from build123d import *

# Parameters (mm, degrees)
SKETCH1_R                       = 19.5
BOSS_EXTRUDE1_DEPTH             = 42
SKETCH2_R                       = 4.75
CUT_EXTRUDE1_DEPTH              = 3
BOSS_EXTRUDE2_DEPTH             = 22
TAP_DRILL_FOR_M4X0_7_TAP1_D     = 3.3
TAP_DRILL_FOR_M4X0_7_TAP1_DEPTH = 10.0000054
TAP_DRILL_FOR_M4X0_7_TAP1_TIP   = 0.991420021
SKETCH6_R                       = 3.5
CUT_EXTRUDE2_DEPTH              = 1.33


with BuildPart() as part:
    # Sketch1 → Boss-Extrude1 (new, symmetric)
    with BuildSketch(Plane(origin=(0, 0, 0), x_dir=(0, 0, -1), z_dir=(1, 0, 0))):
        with Locations(Location((0, 0, 0), (0, 0, 180))):
            Circle(SKETCH1_R)
    extrude(amount=BOSS_EXTRUDE1_DEPTH, both=True)

    # Sketch2 → Cut-Extrude1 (cut)
    with BuildSketch(Plane(origin=(42, 0, 0), x_dir=(0, 0, -1), z_dir=(1, 0, 0))):
        Circle(SKETCH2_R)
    extrude(amount=-CUT_EXTRUDE1_DEPTH, mode=Mode.SUBTRACT)

    # Sketch3 → Boss-Extrude2 (add)
    with BuildSketch(Plane(origin=(39, 0, 0), x_dir=(0, 0, -1), z_dir=(1, 0, 0))):
        with BuildLine():
            Line((-1.486573241, 2.01), (1.486573241, 2.01))
            ThreePointArc((1.486573241, 2.01), (0, -2.5), (-1.486573241, 2.01))
        make_face()
    extrude(amount=BOSS_EXTRUDE2_DEPTH)

    # Tap Drill for M4x0.7 Tap1
    with Locations(Plane(origin=(42, 0, 0), x_dir=(0, 0, -1), z_dir=(1, 0, 0))):
        with Locations((0, 12.5), (12.5, 0), (0, -12.5), (-12.5, 0)):
            Hole(TAP_DRILL_FOR_M4X0_7_TAP1_D / 2, depth=TAP_DRILL_FOR_M4X0_7_TAP1_DEPTH)
            with Locations((0, 0, -(TAP_DRILL_FOR_M4X0_7_TAP1_DEPTH + TAP_DRILL_FOR_M4X0_7_TAP1_TIP / 2))):  # 118° drill point
                Cone(0, TAP_DRILL_FOR_M4X0_7_TAP1_D / 2, TAP_DRILL_FOR_M4X0_7_TAP1_TIP, mode=Mode.SUBTRACT)

    # Sketch6 → Cut-Extrude2 (cut)
    with BuildSketch(Plane.ZY.offset(42)):
        Circle(SKETCH6_R)
        with BuildLine():
            Line((-2.185, 17.03), (2.185, 17.03))
            ThreePointArc((2.185, 17.03), (5.755, 13.46), (2.185, 9.89))
            Line((2.185, 9.89), (-2.185, 9.89))
            ThreePointArc((-2.185, 9.89), (-5.755, 13.46), (-2.185, 17.03))
        make_face()
    extrude(amount=-CUT_EXTRUDE2_DEPTH, mode=Mode.SUBTRACT)


solid = part.part
Read the model definition and answer for the solid it produces. Units are mm, in the model's axes. A direction names the side the tool comes from. Round coordinates to 2 decimals unless told otherwise and drop trailing zeros. Write each loop counter-clockwise with the first axis right and the second up, starting at its lowest first coordinate (ties: lowest second). Pieces come first, ordered by that corner, then holes.
Q1. The mould has two halves that part along Z. Classify faces 1 (the face through (-41.344, -1.341, 3.233)), 2 (the face through (-42, 0, 4)), 3 (the face through (0.588, -19.334, -2.539)): released by +Z, released by -Z, zero draft, split by the parting line, or undercut.
Values:
face 1: undercut
face 2: zero draft
face 3: split by the parting line
Q2. Find section B-B on x = -4.5. Determine the outline of the cut face in (y, z).
Values:
outline: circle Ø39 at (0, 0)
Q3. Straight lines are drawn through the part: line 1 (Y direction, x = -41.2, z = 0); line 2 (Y direction, x = 40.6, z = 0); line 3 (X direction, y = -14, z = 5.5). For each, find the intervals that lie inside material, in ascending order.
Values:
line 1: y = -19.5 to -3.5, 3.5 to 9.89, 17.03 to 19.5
line 2: y = -19.5 to -14.15, -10.85 to -4.75, -2.5 to 2.01, 4.75 to 10.85, 14.15 to 19.5
line 3: x = -42 to 42
Q4. Find section C-C on y = -6.5. Determine the outline of the cut face in (x, z), and give its area (3 significant figures).
Values:
outline: (-42, -18.38) - (42, -18.38) - (42, 18.38) - (-42, 18.38) - close
area: 3,090 mm2
Q5. Flat-ended cylindrical pins translate along their axes: P1, Ø4, axis at y = 0, z = -12.5, coming from the +X side; P2, Ø4, axis at y = 0, z = 0, coming from the -X side; P3, Ø4, axis at x = 38, y = -6, coming from the +Z side. Find the tip coordinate at first contact, or state that the pin passes through.
Values:
P1: stops at x = 42
P2: stops at x = -40.67
P3: stops at z = 19.09
Q6. Find section A-A on x = 34.5. Determine the outline of the cut face in (y, z), and give its area (3 significant figures).
Values:
outline: circle Ø39 at (0, 0); hole circle Ø3.3 at (-12.5, 0); hole circle Ø3.3 at (0, -12.5); hole circle Ø3.3 at (0, 12.5); hole circle Ø3.3 at (12.5, 0)
area: 1,160 mm2
Q7. A tool of negligible diameter and unlimited length cuts with its end or side. For faces 4 (the face through (39, 2.2, 0.1)), 5 (the face through (-40.67, 0, 0)), 6 (the face through (61, 0, 0)), from which of +Z, -Z, +X, -X, +Y, -Y can it reach the whole face along a straight path? Write none if from no direction.
Values:
face 4: +X
face 5: -X
face 6: +Z, -Z, +X, +Y, -Y
